Solid Edge part; units mm, degrees
sketch "Sketch1" plane through (0, 0, 0) normal (0, 0, 1) x (1, 0, 0)
  circle A0 centre (0, 0) radius 7
  circle A1 centre (0, 0) radius 3.175
extrude "Protrusion1" add sketch "Sketch1" along normal blind 25
fillet "Round_1" radius 0.5 4 edges at (-7, 0, 25) (-7, 0, 0) (-3.175, 0, 0) (-3.175, 0, 25)
sketch "Sketch2" plane through (0, 0, 25) normal (0, 0, 1) x (1, 0, 0)
  circle A0 centre (0, 0) radius 4
extrude "ExtrudedCutout_1" cut sketch "Sketch2" against normal blind 12
fillet "Round_2" radius 0.5 1 edges at (-4, 0, 25)
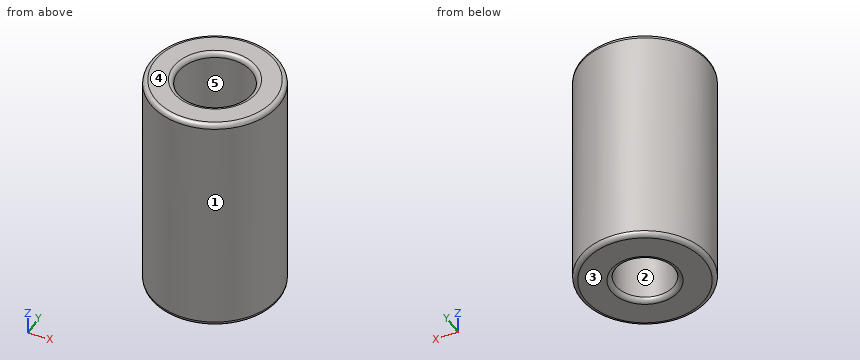
The listing builds one solid part. Answer for the finished solid, in the listing's coordinates (mm). Face numbers are marked on the shaded views. A direction names the side the tool comes from. Round coordinates to 2 decimals unless told otherwise and drop trailing zeros. Write each loop counter-clockwise with the first axis right and the second up, starting at its lowest first coordinate (ties: lowest second). Pieces come first, ordered by that corner, then holes. Notation, with made-up numbers: (85, 10) -> (141, 10) arc R23 cw to (141, 32) -> close; hole circle Ø8 at (62, -22.5). An arc over 180 degrees is marked (long way). Use CSV: the item, a comma, the result in double quotes. Start each with the question number.
(1) Which of the six approach directions +Z, -Z, +X, -X, +Y, -Y give full straight-line access (tool end or side, diameter ignored) to the marked faces 4 and 5?
(2) Each of these flat-tipped pins is pushed along its axis until it touches: pin 1 (5 mm diameter, centred on x = -1, z = 12.5, fed in from +Y); pin 2 (8 mm diameter, centred on x = -4.5, z = 7, fed in from -Y); pin 3 (4 mm diameter, centred on x = 0, y = -1.5, fed in from +Z); pin 4 (1.5 mm diameter, centred on x = 3.5, y = -1, fed in from +Z). Where does it stop, or does it pass through?
(3) Consider L1, parallel to Y at x = 0, z = 3 (3 decimals); L2, parallel to Y at x = 0, z = 16.25; L3, parallel to X at y = 3.5, z = 14. Determine where each line is inside the solid, lowest interval first. Write a range as from..to.
(4) Section A-A on x = 0 is taken. Give the vertices of the cut face in (y, z) (3 decimals).
(5) Section C-C on z = 23.5 is taken. Give the vertices of the cut face in (x, y).
(6) The mould has two halves that part along Y. Classify the marked faces 1, 2 and 3: released by +Y, released by -Y, zero draft, split by the parting line, or undercut.
A:
1,face 4,"+Z, +X, -X, +Y, -Y"
1,face 5,"+Z"
2,pin 1,"stops at y = 7"
2,pin 2,"stops at y = -6.98"
2,pin 3,"stops at z = 13"
2,pin 4,"stops at z = 24.99"
3,L1,"y = -7..-3.175, 3.175..7"
3,L2,"y = -7..-4, 4..7"
3,L3,"x = -6.06..-1.94, 1.94..6.06"
4,outline,"(-7, 0.5) arc R0.5 ccw to (-6.5, 0) -> (-3.675, 0) arc R0.5 ccw to (-3.175, 0.5) -> (-3.175, 13) -> (-4, 13) -> (-4, 24.5) arc R0.5 ccw to (-4.5, 25) -> (-6.5, 25) arc R0.5 ccw to (-7, 24.5) -> close; (3.175, 0.5) arc R0.5 ccw to (3.675, 0) -> (6.5, 0) arc R0.5 ccw to (7, 0.5) -> (7, 24.5) arc R0.5 ccw to (6.5, 25) -> (4.5, 25) arc R0.5 ccw to (4, 24.5) -> (4, 13) -> (3.175, 13) -> close"
5,outline,"circle Ø14 at (0, 0); hole circle Ø8 at (0, 0)"
6,face 1,"split by the parting line"
6,face 2,"undercut"
6,face 3,"zero draft"
